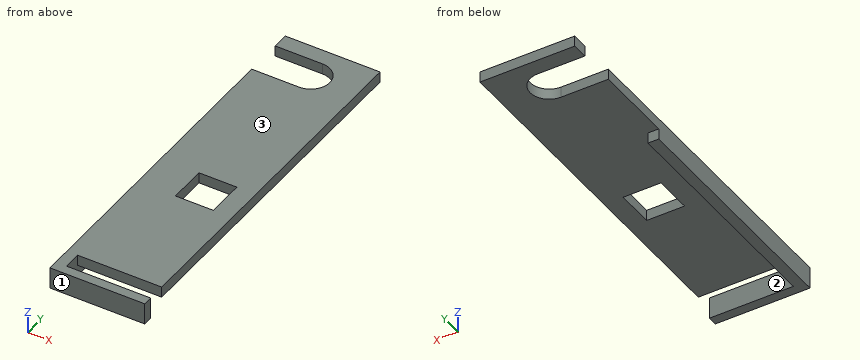
```python
from build123d import *

# Parameters (mm, degrees)
F0_W     = 14
F0_H     = 14
F1_DEPTH = 4
F2_W     = 31
F2_H     = 3.5
F3_DEPTH = 4


with BuildPart() as f1:
    # F0 (on Top) → F1 (new body)
    with BuildSketch(Plane.XY):
        with BuildLine():
            Line((17.5, -59.9), (17.5, 70))
            Line((17.5, 70), (-17.5, 70))
            Line((-17.5, 70), (-17.5, 64))
            Line((-17.5, 64), (0, 64))
            ThreePointArc((0, 64), (7, 57), (0, 50))
            Line((0, 50), (-17.5, 50))
            Line((-17.5, 50), (-17.5, -70))
            Line((-17.5, -70), (17.5, -70))
            Line((17.5, -70), (17.5, -66.5))
            Line((17.5, -66.5), (-13.5, -66.5))
            Line((-13.5, -66.5), (-13.5, -59.9))
            Line((-13.5, -59.9), (17.5, -59.9))
        make_face()
        with Locations((3.5, -10.9)):
            Rectangle(F0_W, F0_H, mode=Mode.SUBTRACT)
    extrude(amount=F1_DEPTH)

    # F2 (on face) → F3 (join)
    with BuildSketch(Plane(origin=(0, 0, 0), x_dir=(1, 0, 0), z_dir=(0, 0, -1))):
        Polygon((-13.5, 70), (-17.5, 70), (-17.5, -20), (-13.5, -20), (-13.5, 66.5), align=None)
        with Locations((2, 68.25)):
            Rectangle(F2_W, F2_H)
    extrude(amount=F3_DEPTH)


solid = f1.part
```
For this review, take the finished solid that the model builds, in its own axes (mm). Face numbers are marked on the shaded views. Coordinates: 2 decimals unless noted, no trailing zeros. Write each loop counter-clockwise with the first axis right and the second up, starting at its lowest first coordinate (ties: lowest second). Pieces come first, ordered by that corner, then holes. Notation, with made-up numbers: (-32.5, 40) - (24.5, 40) arc R19 cw to (24.5, 62) - close; hole circle Ø7 at (87, -29.5). An arc over 180 degrees is marked (long way). Answer in a Markdown table with one row per item. Add a question column.
Q1. For P1, Ø3, axis at x = -9, z = -1, coming from the +Y side; P2, Ø17.5, axis at x = -1, y = 15, coming from the -Z side, all flat-tipped, find the tip position at first contact; note any pin that passes through.
Q2. We need section B-B, the plane z = 1.25. State the section outline as (x, y) points, and give its area (3 significant figures).
Q3. For probe 1 along Y at (x, z) = (8.5, 3.75); probe 2 along Y at (x, z) = (-5, 3.25); probe 3 along Y at (x, z) = (-14.5, 2.75), list the stretches that pass through material, from the lowest coordinate up.
Q4. We need section D-D, the plane y = 57. State the section outline as (x, z) points, and give its area (3 significant figures).
Q5. Draft analysis for pull direction Y (two halves, no side actions). For the marked faces 1, 2 and 3, state which applies: +Y half, -Y half, draft (parallel to the pull), parting line (faces both ways), or undercut.
Q6. We need section A-A, the plane x = -15. State the section outline as (y, z) points.
Q7. We need section C-C, the plane x = -6.5. State the section outline as (y, z) points.
Answer list:
| question | item | result |
|---|---|---|
| 1 | P1 | stops at y = 70 |
| 1 | P2 | stops at z = 0 |
| 2 | outline | (-17.5, -70) - (17.5, -70) - (17.5, -66.5) - (-13.5, -66.5) - (-13.5, -59.9) - (17.5, -59.9) - (17.5, 70) - (-17.5, 70) - (-17.5, 64) - (0, 64) arc R7 cw to (0, 50) - (-17.5, 50) - close; hole (-3.5, -17.9) - (10.5, -17.9) - (10.5, -3.9) - (-3.5, -3.9) - close |
| 2 | area | 4,180 mm2 |
| 3 | probe 1 | y = -70 to -66.5, -59.9 to -17.9, -3.9 to 70 |
| 3 | probe 2 | y = -70 to -66.5, -59.9 to 50, 64 to 70 |
| 3 | probe 3 | y = -70 to 50, 64 to 70 |
| 4 | outline | (7, 0) - (17.5, 0) - (17.5, 4) - (7, 4) - close |
| 4 | area | 42.0 mm2 |
| 5 | face 1 | -Y half |
| 5 | face 2 | undercut |
| 5 | face 3 | draft |
| 6 | outline | (-70, -4) - (20, -4) - (20, 0) - (50, 0) - (50, 4) - (-70, 4) - close; (64, 0) - (70, 0) - (70, 4) - (64, 4) - close |
| 7 | outline | (-70, -4) - (-66.5, -4) - (-66.5, 4) - (-70, 4) - close; (-59.9, 0) - (50, 0) - (50, 4) - (-59.9, 4) - close; (64, 0) - (70, 0) - (70, 4) - (64, 4) - close |
